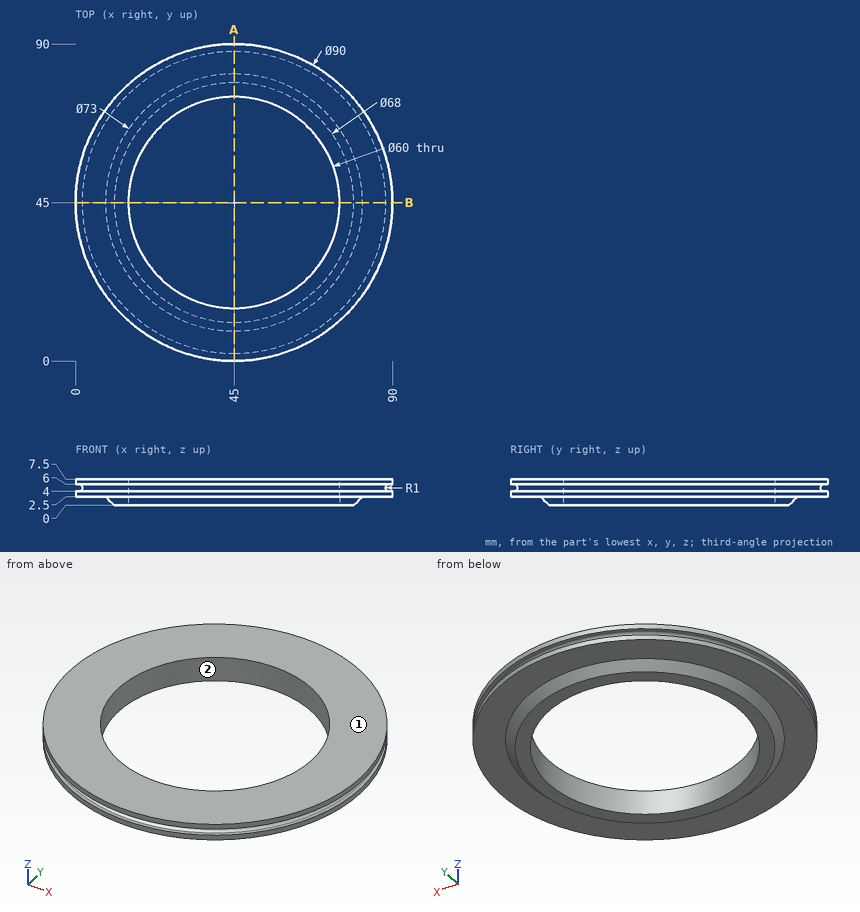
Study the drawing (mm; zero at the part's minimum x, y, z) and answer. Coordinates: 2 decimals unless noted, no trailing zeros. Order: outer loops, then holes, each group sorted by start corner. A loop starts at its lowest first (then second) coordinate and runs counter-clockwise, first axis right, second up. Notation, with made-up numbers: M -3,8 L 26,8 A21 ccw 26,27 Z; hole C 32,-11.75 d5. An arc over 180 degrees is marked long. Answer as a JSON object with one key per item and string values. Group by question number.
1. Flat-ended cylindrical pins translate along their axes: P1, Ø4, axis at y = 72.5, z = 3, coming from the +X side; P2, Ø1, axis at x = 40, z = 1, coming from the +Y side; P3, Ø1, axis at y = 31.5, z = 2.5, coming from the +X side. Find the tip coordinate at first contact, or state that the pin passes through.
2. Determine the mould class of the marked faces 1 and 2 for opening direction X: released by +X, released by -X, zero draft, split by the parting line, or undercut.
3. Section A-A on x = 45 is taken. Write down the section's boundary in (y, z), then the cut area to 3 significant figures.
4. Straight lines are drawn through the part: line 1 (X direction, y = 45, z = 3.25); line 2 (Z direction, x = 60, y = 83.5); line 3 (Y direction, x = 44.5, z = 4.5). For each, find the intervals that lie inside material, in ascending order.
Values follow:
{
 "1": {"P1": "x = 82.08", "P2": "y = 80.15", "P3": "x = 88.08"},
 "2": {"face 1": "zero draft", "face 2": "undercut"},
 "3": {"outline": "M 0,2.5 L 8.5,2.5 L 11,0 L 15,0 L 15,7.5 L 0,7.5 L 0,6 L 1,6 A1 cw 1,4 L 0,4 Z; M 75,0 L 79,0 L 81.5,2.5 L 90,2.5 L 90,4 L 89,4 A1 cw 89,6 L 90,6 L 90,7.5 L 75,7.5 Z", "area": "169 mm2"},
 "4": {"line 1": "0 to 15, 75 to 90", "line 2": "2.5 to 7.5", "line 3": "1.87 to 15, 75 to 88.13"}
}
